Drawing for the job (mm, zero at the part's lowest x, y, z). Round coordinates to 2 decimals unless told otherwise and drop trailing zeros. Write each loop counter-clockwise with the first axis right and the second up, starting at its lowest first coordinate (ties: lowest second). Pieces come first, ordered by that corner, then holes.
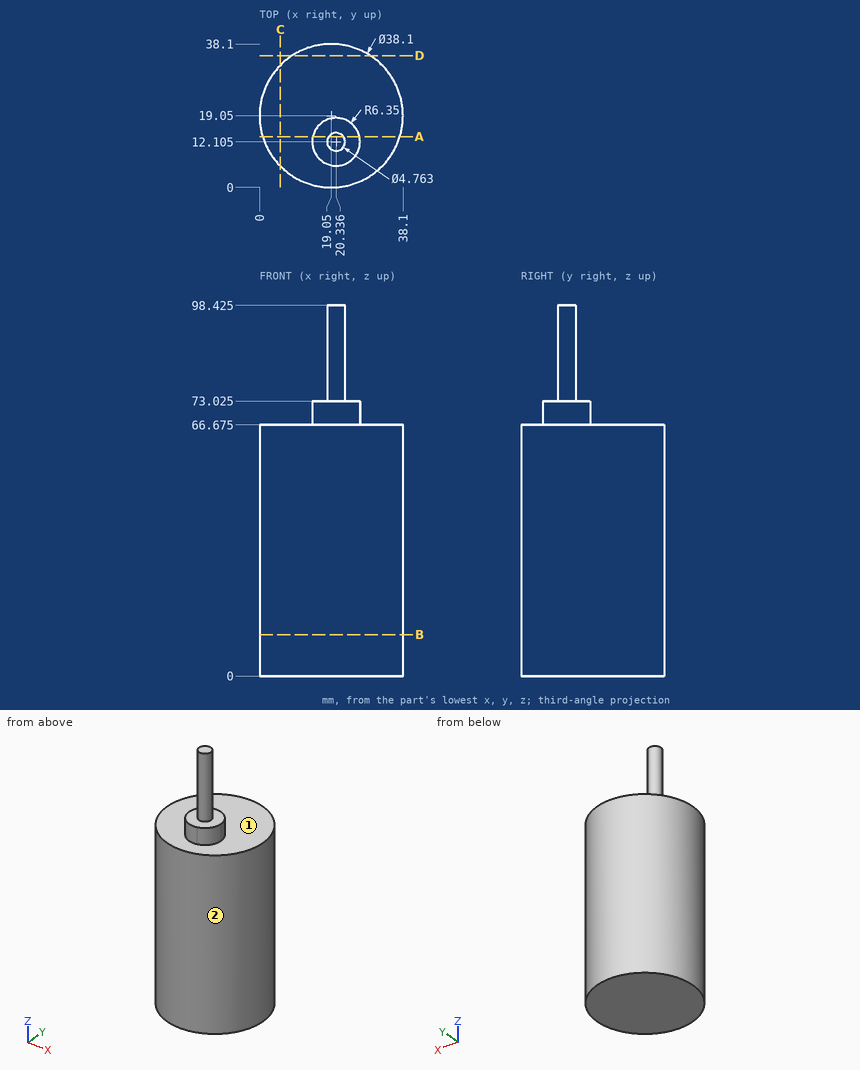
1) Cut at B-B on z = 11. List the corners of the cut face in (x, y), and give its area (3 significant figures).
2) Cut at C-C on x = 5.5. List the corners of the cut face in (y, z) (1 decimal), and give its area (3 significant figures).
3) Flat gauge pins, fed straight in: pin 1 Ø12 at (x, z) = (10.5, 53) entering from -Y; pin 2 Ø6 at (x, y) = (5, 4.5) entering from +Z (1 decimal); pin 3 Ø4 at (y, z) = (10, 72) entering from -X. Where does each tip first touch, or does it go through?
4) Cut at A-A on y = 13.5. List the corners of the cut face in (x, z) (1 decimal), and give its area (3 significant figures).
5) Pull direction X, two halves, no side cores. Call the marked faces 1 and 2: released by +X, released by -X, zero draft, split by the parting line, or undercut.
6) Cut at D-D on y = 35. List the corners of the cut face in (x, z) (1 decimal).
7) Wall check: probe 1 along Z at (x, y) = (18, 33.5) (1 decimal); probe 2 along Z at (x, y) = (19.5, 7.5) (1 decimal); probe 3 along Y at (x, z) = (18.5, 51.5). Give the ranges that are in metal, low to high.
Result sheet:
1. outline: circle Ø38.1 at (19.05, 19.05)
1. area: 1,140 mm2
2. outline: (5.7, 0) - (32.4, 0) - (32.4, 66.7) - (5.7, 66.7) - close
2. area: 1,790 mm2
3. pin 1: stops at y = 0.17
3. pin 2: stops at z = 66.7
3. pin 3: stops at x = 13.99
4. outline: (0.8, 0) - (37.3, 0) - (37.3, 66.7) - (26.5, 66.7) - (26.5, 73) - (22.3, 73) - (22.3, 98.4) - (18.4, 98.4) - (18.4, 73) - (14.1, 73) - (14.1, 66.7) - (0.8, 66.7) - close
4. area: 2,610 mm2
5. face 1: zero draft
5. face 2: split by the parting line
6. outline: (8.6, 0) - (29.5, 0) - (29.5, 66.7) - (8.6, 66.7) - close
7. probe 1: z = 0 to 66.7
7. probe 2: z = 0 to 73
7. probe 3: y = 0.01 to 38.09
